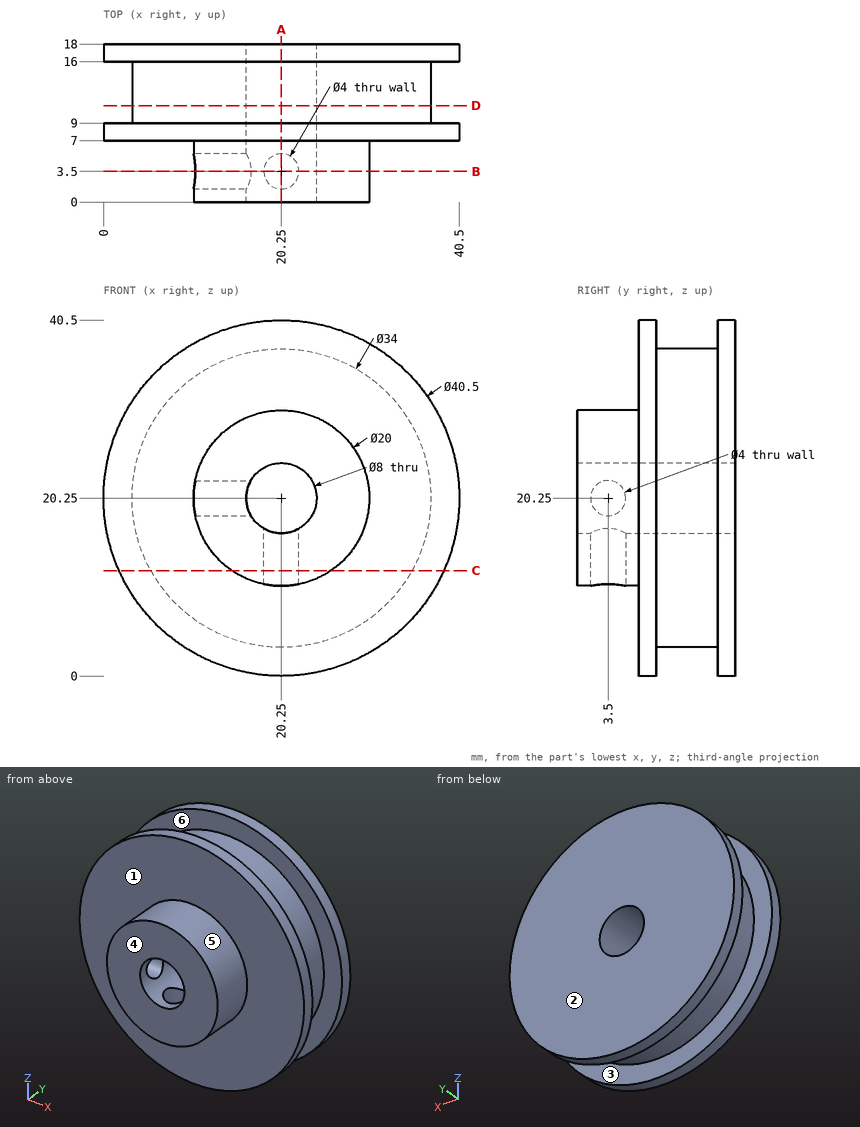
Check sheet for the drawn part. Datum: minimum x, y, z corner. Units: mm. A direction names the side the tool comes from. Give positions to 0.01 mm unless a question says otherwise; leave off trailing zeros. Order: outer loops, then holes, each group sorted by start corner. A loop starts at its lowest first (then second) coordinate and runs counter-clockwise, first axis right, second up. Notation, with made-up numbers: (66, -18) -> (85, -18) arc R21 ccw to (85, -6) -> close; hole circle Ø3 at (73, 13). An arc over 180 degrees is marked (long way). Use a Markdown table: item, result.
1) Section check D-D, the plane y = 11. Record the boundary of the cut face in (x, z), then the cut area to 3 significant figures.
Results:
| item | result |
|---|---|
| outline | circle Ø34 at (20.25, 20.25); hole circle Ø8 at (20.25, 20.25) |
| area | 858 mm² |
2) Section check A-A, the plane x = 20.25. Record the boundary of the cut face in (y, z).
Results:
| item | result |
|---|---|
| outline | (0, 10.25) -> (1.5, 10.25) -> (1.5, 16.25) -> (0, 16.25) -> close; (0, 24.25) -> (18, 24.25) -> (18, 40.5) -> (16, 40.5) -> (16, 37.25) -> (9, 37.25) -> (9, 40.5) -> (7, 40.5) -> (7, 30.25) -> (0, 30.25) -> close; (5.5, 10.25) -> (7, 10.25) -> (7, 0) -> (9, 0) -> (9, 3.25) -> (16, 3.25) -> (16, 0) -> (18, 0) -> (18, 16.25) -> (5.5, 16.25) -> close |
3) Section check C-C, the plane z = 12. Record the boundary of the cut face in (x, y), then the cut area to 3 significant figures.
Results:
| item | result |
|---|---|
| outline | (1.76, 7) -> (14.6, 7) -> (14.6, 0) -> (25.9, 0) -> (25.9, 7) -> (38.74, 7) -> (38.74, 9) -> (35.11, 9) -> (35.11, 16) -> (38.74, 16) -> (38.74, 18) -> (1.76, 18) -> (1.76, 16) -> (5.39, 16) -> (5.39, 9) -> (1.76, 9) -> close; hole circle Ø4 at (20.25, 3.5) |
| area | 423 mm² |
4) Depth check by flat-ended pin: pin 1 Ø2.5 at (x, y) = (20.25, 3.5) entering from -Z; pin 2 Ø1.5 at (y, z) = (5.5, 24.5) entering from +X; pin 3 Ø3 at (y, z) = (3.5, 20.25) entering from -X; pin 4 Ø6.5 at (x, z) = (20.25, 20.25) entering from -Y. Enter the tip coordinate at first touch or a pass-through.
Results:
| item | result |
|---|---|
| pin 1 | z = 24.05 |
| pin 2 | x = 29.62 |
| pin 3 | x = 23.96 |
| pin 4 | through |
5) Tool access check on the marked faces 4, 5 and 6. Record the directions out of +Z, -Z, +X, -X, +Y, -Y that give a thin tool (end or side, any length) a straight path to the whole face; none if there is none.
Results:
| item | result |
|---|---|
| face 4 | +Z, -Z, +X, -X, -Y |
| face 5 | -Y |
| face 6 | none |
6) Section check B-B, the plane y = 3.5. Record the boundary of the cut face in (x, z), then the cut area to 3 significant figures.
Results:
| item | result |
|---|---|
| outline | (10.45, 18.25) arc R10 ccw to (18.25, 10.45) -> (18.25, 16.79) arc R4 cw to (16.79, 18.25) -> close; (10.45, 22.25) -> (16.79, 22.25) arc R4 cw (long way) to (22.25, 16.79) -> (22.25, 10.45) arc R10 ccw (long way) to start |
| area | 215 mm² |
7) Mould release check, pull along Y, two halves, no side actions. Record for the marked faces 1, 2 and 3: pulls with the +Y half, pulls with the -Y half, needs draft (parallel to the pull), parting line crosses it, or undercut.
Results:
| item | result |
|---|---|
| face 1 | pulls with the -Y half |
| face 2 | pulls with the +Y half |
| face 3 | undercut |
8) Material ranges on probe 1 along Y at (x, z) = (7.5, 32.5); probe 2 along X at (y, z) = (6.25, 20.25); probe 3 along X at (y, z) = (12.25, 20.25), recorded low to high.
Results:
| item | result |
|---|---|
| probe 1 | 7 to 9, 16 to 18 |
| probe 2 | 10.25 to 16.25, 24.25 to 30.25 |
| probe 3 | 3.25 to 16.25, 24.25 to 37.25 |
